Build history of the part. All positions in model axes, mm. Face numbers are marked on the shaded views. A direction names the side the tool comes from. Round coordinates to 2 decimals unless told otherwise and drop trailing zeros. Write each loop counter-clockwise with the first axis right and the second up, starting at its lowest first coordinate (ties: lowest second). Pieces come first, ordered by that corner, then holes.
1) Flat gauge pins, fed straight in: pin 1 (4.5 mm diameter, centred on y = 40.5, z = 4, fed in from -X); pin 2 (20 mm diameter, centred on x = 23, z = 33, fed in from +Y); pin 3 (12 mm diameter, centred on y = -59.5, z = 18, fed in from -X). Where does each tip first touch, or does it go through?
2) Saw through at A-A (y = -9.5). Write the cut outline in (x, z).
3) Pull direction X, two halves, no side cores. Call the marked faces 1, 2, 3 and 4: +X half, -X half, draft (parallel to the pull), parting line (faces both ways), or undercut.
4) Wall check: probe 1 along Z at (x, y) = (25, -55); probe 2 along Z at (x, y) = (25, -33); probe 3 along X at (y, z) = (0, 5). Give the ranges that are in metal, low to high.
5) Saw through at D-D (x = 87). Write the cut outline in (y, z), plus the area to 3 significant figures.
6) Saw through at B-B (x = 25). Write the cut outline in (y, z), plus the area to 3 significant figures.
7) Which spindle directions (+Z, -Z, +X, -X, +Y, -Y) get a long thin tool onto all of the face, cutting with end or side? Do the marked faces 5, 6 and 7. Say none if no direction does.
8) Saw through at C-C (y = -54). Write the cut outline in (x, z).
from build123d import *

# Parameters (mm, degrees)
PAD_DEPTH    = 10
PAD001_DEPTH = 22
SKETCH003_W  = 17
SKETCH003_H  = 7
PAD002_DEPTH = 50
FILLET_R     = 6
FILLET001_R  = 5
FILLET002_R  = 5
SKETCH004_R  = 2.5
POCKET_DEPTH = 10.001
SKETCH005_R  = 11
PAD003_DEPTH = 30
SKETCH006_R  = 11
PAD004_DEPTH = 5
PAD005_DEPTH = 9
SKETCH008_W  = 22.5
SKETCH008_H  = 2
PAD006_DEPTH = 3


with BuildPart() as part:
    # Sketch → Pad (new body)
    with BuildSketch(Plane.XY):
        with BuildLine():
            Line((123, 46.5), (0, 46.5))
            Line((0, 46.5), (0, -35.5))
            Line((0, -35.5), (40, -35.5))
            Line((40, -35.5), (40, -25.5))
            Line((40, -25.5), (10, -25.5))
            Line((10, -25.5), (10, 41.5))
            Line((10, 41.5), (123, 41.5))
            Line((123, 41.5), (123, 37.5))
            Line((123, 37.5), (127, 41.5))
            Line((127, 41.5), (127, 42.5))
            ThreePointArc((127, 42.5), (125.828427, 45.328427), (123, 46.5))
        make_face()
    extrude(amount=PAD_DEPTH)

    # Sketch002 (on Face13 of Pad) → Pad001 (join)
    with BuildSketch(Plane.XY.offset(10)):
        Polygon((0, -35.5), (40, -35.5), (40, -25.5), (10, -25.5), (10, 17), (0, 17), align=None)
    extrude(amount=PAD001_DEPTH)

    # Sketch003 (on Face20 of Pad001) → Pad002 (join)
    with BuildSketch(Plane.YZ.offset(10)):
        with Locations((8.5, 28.5)):
            Rectangle(SKETCH003_W, SKETCH003_H)
    extrude(amount=PAD002_DEPTH)

    # Fillet
    fillet_edges = [part.edges().sort_by_distance(p)[0] for p in [
        (60, 8.5, 32),
    ]]
    fillet(fillet_edges, radius=FILLET_R)

    # Fillet001
    fillet001_edges = [part.edges().sort_by_distance(p)[0] for p in [
        (0, 46.5, 5),
    ]]
    fillet(fillet001_edges, radius=FILLET001_R)

    # Fillet002
    fillet002_edges = [part.edges().sort_by_distance(p)[0] for p in [
        (0, -9.25, 32),
    ]]
    fillet(fillet002_edges, radius=FILLET002_R)

    # Sketch004 (on Face19 of Fillet002) → Pocket (cut, through all)
    with BuildSketch(Plane(origin=(0, -25.5, 0), x_dir=(-1, 0, 0), z_dir=(0, 1, 0))):
        with Locations((-25, 16)):
            Circle(SKETCH004_R)
    extrude(amount=-POCKET_DEPTH, mode=Mode.SUBTRACT)

    # Sketch005 (on Face9 of Pocket) → Pad003 (join)
    with BuildSketch(Plane.XZ.offset(35.5)):
        with BuildLine():
            ThreePointArc((40, 16), (25, 31), (10, 16))
            Line((10, 16), (10, 0))
            Line((10, 0), (40, 0))
            Line((40, 0), (40, 16))
        make_face()
        with Locations((25, 16)):
            Circle(SKETCH005_R, mode=Mode.SUBTRACT)
    extrude(amount=PAD003_DEPTH)

    # Sketch006 (on Face34 of Pad003) → Pad004 (join)
    with BuildSketch(Plane.XZ.offset(65.5)):
        with BuildLine():
            ThreePointArc((40, 26), (25, 41), (10, 26))
            Line((10, 11), (10, 26))
            Line((10, 11), (-12.5, 11))
            Line((-12.5, 11), (-12.5, 0))
            Line((-12.5, 0), (62.5, 0))
            Line((62.5, 0), (62.5, 11))
            Line((62.5, 11), (40, 11))
            Line((40, 11), (40, 26))
        make_face()
        with Locations((25, 16)):
            Circle(SKETCH006_R, mode=Mode.SUBTRACT)
    extrude(amount=PAD004_DEPTH)

    # Sketch007 (on Face40 of Pad004) → Pad005 (join)
    with BuildSketch(Plane(origin=(0, 0, 0), x_dir=(1, 0, 0), z_dir=(0, 0, -1))):
        with BuildLine():
            Line((52.5, 70.5), (52.5, 94))
            Line((52.5, 94), (-9.5, 94))
            ThreePointArc((-9.5, 94), (-11.62132, 93.12132), (-12.5, 91))
            Line((-12.5, 91), (-13.5, 91))
            Line((-13.5, 91), (-13.5, 99))
            Line((62.5, 104), (-13.5, 99))
            Line((62.5, 104), (62.5, 94))
            Line((62.5, 94), (62.5, 70.5))
            Line((62.5, 70.5), (52.5, 70.5))
        make_face()
    extrude(amount=-PAD005_DEPTH)

    # Sketch008 (on Face43 of Pad005) → Pad006 (join)
    with BuildSketch(Plane.XZ.offset(70.5)):
        with Locations((51.25, 10)):
            Rectangle(SKETCH008_W, SKETCH008_H)
        with Locations((-1.25, 10)):
            Rectangle(SKETCH008_W, SKETCH008_H)
    extrude(amount=PAD006_DEPTH)


solid = part.part
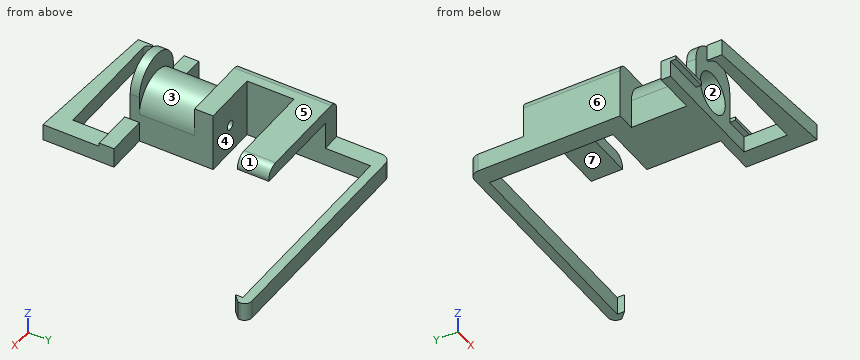
Evaluation:
1. pin 1: stops at x = 0
1. pin 2: stops at y = 17
1. pin 3: stops at x = 10
2. outline: (0, 0) - (10, 0) - (10, 32) - (5, 32) arc R5 ccw to (0, 27) - close
3. face 1: +X half
3. face 2: undercut
3. face 3: parting line
3. face 4: draft
4. probe 1: z = 0 to 5, 27 to 31
4. probe 2: z = 0 to 13.5, 18.5 to 32
4. probe 3: x = 0 to 10
5. outline: (41.5, 0) - (46.5, 0) - (46.5, 10) - (41.5, 10) - close
5. area: 50.0 mm2
6. outline: (-101.53, 0) - (-94, 0) - (-94, 9) - (-101.53, 9) - close; (-70.5, 0) - (-25.5, 0) - (-25.5, 13.5) - (-35.5, 13.5) - (-35.5, 5) - (-70.5, 5) - close; (-70.5, 27) - (-35.5, 27) - (-35.5, 18.5) - (-25.5, 18.5) - (-25.5, 32) - (-35.5, 32) - (-35.5, 31) - (-65.5, 31) - (-65.5, 41) - (-70.5, 41) - close; (0, 25) - (17, 25) - (17, 32) - (0, 32) - close; (41.5, 0) - (46.5, 0) - (46.5, 10) - (41.5, 10) - close
6. area: 872 mm2
7. face 5: +Z, +X, -X, +Y
7. face 6: +Z, -Z, -X, +Y
7. face 7: -Z, +X, +Y
8. outline: (10, 0) - (40, 0) - (40, 16) arc R15 ccw to (10, 16) - close; hole circle Ø22 at (25, 16)
